```python
from build123d import *

# Parameters (mm, degrees)
SKETCH_1_R          = 6
EXTRUDE_1_DEPTH     = 70
SKETCH_2_W          = 10
SKETCH_2_H          = 1
SKETCH_2_W_2        = 20
CUT_EXTRUDE_1_DEPTH = 35
EXTRUDE_2_DEPTH     = 10


with BuildPart() as part:
    # 草图1 → 凸台-拉伸1 (new body)
    with BuildSketch(Plane(origin=(0, 0, 0), x_dir=(0, 0, -1), z_dir=(1, 0, 0))):
        Circle(SKETCH_1_R)
    extrude(amount=EXTRUDE_1_DEPTH)

    # 草图2 → 切除-拉伸1 (cut, symmetric)
    with BuildSketch(Plane.XY):
        with Locations((55, 5.5)):
            Rectangle(SKETCH_2_W, SKETCH_2_H)
        with Locations((10, 5.5)):
            Rectangle(SKETCH_2_W_2, SKETCH_2_H)
    extrude(amount=CUT_EXTRUDE_1_DEPTH, both=True, mode=Mode.SUBTRACT)

    # 草图3 → 凸台-拉伸2 (add)
    with BuildSketch(Plane.ZY):
        with BuildLine():
            Line((-3.31662479, 5), (3.31662479, 5))
            ThreePointArc((3.31662479, 5), (0, -6), (-3.31662479, 5))
        make_face()
    extrude(amount=EXTRUDE_2_DEPTH)


solid = part.part
```
Geometry: final body of the model. Coordinates: model frame, mm. A direction names the side the tool comes from. Round coordinates to 2 decimals unless told otherwise and drop trailing zeros. Write each loop counter-clockwise with the first axis right and the second up, starting at its lowest first coordinate (ties: lowest second). Pieces come first, ordered by that corner, then holes. Notation, with made-up numbers: (2.5, 78) -> (43.5, 78) arc R24 ccw to (43.5, 104) -> close; hole circle Ø5 at (21.5, -13.75). An arc over 180 degrees is marked (long way). Return JSON: item names as keys, results as strings.
Q1. First-contact query: pin 1 Ø2 at (x, z) = (8.5, 3.5) entering from +Y; pin 2 Ø2 at (x, z) = (24.5, 1) entering from -Y; pin 3 Ø0.8 at (y, z) = (5.5, 0) entering from -X; pin 4 Ø3 at (x, z) = (42.5, 2.5) entering from -Y. Flat tips, straight axial feed; report the tip coordinate or a pass-through.
From the geometry:
{"pin 1": "y = 5", "pin 2": "y = -6", "pin 3": "x = 20", "pin 4": "y = -5.92"}
Q2. Section A-A on z = 0. Return the cut outline in (x, y).
From the geometry:
{"outline": "(-10, -6) -> (70, -6) -> (70, 6) -> (60, 6) -> (60, 5) -> (50, 5) -> (50, 6) -> (20, 6) -> (20, 5) -> (-10, 5) -> close"}
Q3. Section D-D on z = 4.75. Return the cut outline in (x, y).
From the geometry:
{"outline": "(-10, -3.67) -> (70, -3.67) -> (70, 3.67) -> (-10, 3.67) -> close"}
Q4. Ray query, line 1 (Y direction, x = 63.5, z = 0.25); line 2 (Y direction, x = 52.5, z = 5). Return the intervals inside material, ascending.
From the geometry:
{"line 1": "-5.99 to 5.99", "line 2": "-3.32 to 3.32"}
Q5. Section C-C on x = 26.5. Return the cut outline in (y, z).
From the geometry:
{"outline": "circle Ø12 at (0, 0)"}
Q6. Set-up query: faces 1 (the flat face through (-10, 0, 0)), 2 (the flat face through (5, 5, 0)), 3 (the flat face through (55, 5, 0)). Return all of +Z, -Z, +X, -X, +Y, -Y with unobstructed straight access to the full face (end or side cutting, diameter ignored); none if empty.
From the geometry:
{"face 1": "+Z, -Z, -X, +Y, -Y", "face 2": "+Z, -Z, -X, +Y", "face 3": "+Z, -Z, +Y"}
Q7. Section B-B on y = -5. Return the cut outline in (x, z), and give its area (3 significant figures).
From the geometry:
{"outline": "(-10, -3.32) -> (70, -3.32) -> (70, 3.32) -> (-10, 3.32) -> close", "area": "531 mm2"}
